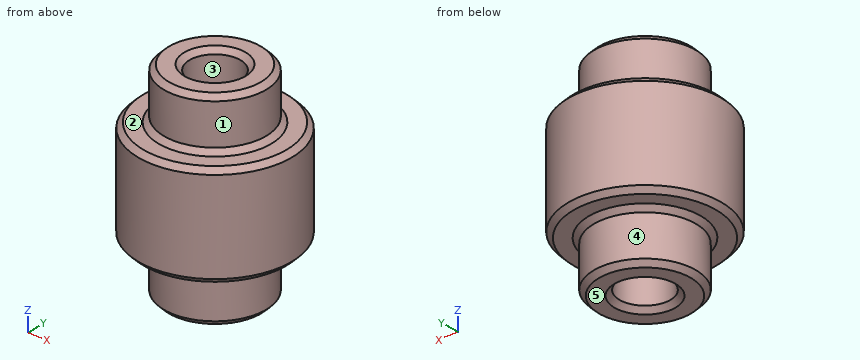
```python
from build123d import *

# Parameters (mm, degrees)
F0_R          = 15
F1_DEPTH      = 10
F1_DEPTH_BACK = 10
F2_R          = 10
F3_DEPTH      = 10
F4_R          = 10
F5_DEPTH      = 10
F7_D          = 10
F8_SIZE       = 1


with BuildPart() as f1:
    # F0 (on Top) → F1 (new body, two sides)
    with BuildSketch(Plane.XY) as f1_sk:
        Circle(F0_R)
    extrude(amount=F1_DEPTH)
    extrude(f1_sk.sketch, amount=-F1_DEPTH_BACK)

    # F2 (on face) → F3 (join)
    with BuildSketch(Plane.XY.offset(10)):
        Circle(F2_R)
    extrude(amount=F3_DEPTH)

    # F4 (on face) → F5 (join)
    with BuildSketch(Plane(origin=(0, 0, -10), x_dir=(1, 0, 0), z_dir=(0, 0, -1))):
        Circle(F4_R)
    extrude(amount=F5_DEPTH)

    # F7 (through all)
    with Locations(Plane.XY.offset(20)):
        with Locations((0, 0)):
            Hole(F7_D / 2)

    # F8
    f8_edges = [f1.edges().sort_by_distance(p)[0] for p in [
        (-10, 0, 20),
        (-5, 0, 20),
        (-15, 0, 10),
        (-10, 0, 10),
        (-15, 0, -10),
        (-10, 0, -10),
        (-10, 0, -20),
        (-5, 0, -20),
    ]]
    chamfer(f8_edges, length=F8_SIZE)


solid = f1.part
```
Can you work these out from the model? Positions are in its coordinate system, mm. Face numbers are marked on the shaded views. A direction names the side the tool comes from. Round coordinates to 2 decimals unless told otherwise and drop trailing zeros. Loops run counter-clockwise (first coordinate to the right, second up) from the corner with the lowest first, then second, coordinate; pieces in that order, holes last.
Item 1: Please list where these lines run through material, in increasing order: L1, parallel to Y at x = 0, z = 8; L2, parallel to Z at x = -5.25, y = -11.5; L3, parallel to Y at x = 4, z = 9.
Item 2: If we mould it in two halves opening along X, with no side actions, what happens to the marked faces 1, 2 and 3? For each: +X half, -X half, draft (parallel to the pull), parting line (faces both ways), or undercut.
Item 3: Suppose I cut it at C-C, the plane z = 4. Write out the boundary of the cut face in (x, y).
Item 4: Suppose I cut it at D-D, the plane z = 13. Write out the boundary of the cut face in (x, y), then the cut area to 3 significant figures.
Item 5: Will these pins go through, and if not, where does the flat tip stop? pin 1 Ø1 at (y, z) = (-6, -2.5) entering from +X; pin 2 Ø4 at (y, z) = (4.5, 14) entering from +X; pin 3 Ø4 at (y, z) = (11.5, -6.5) entering from +X.
Item 6: Which directions (+Z, -Z, +X, -X, +Y, -Y) give clear straight access to the entire face, cutting with the end or side of a thin tool? Please do the marked faces 4 and 5.
Reported:
1. L1: y = -15 to -5, 5 to 15
1. L2: z = -10 to 10
1. L3: y = -14.46 to -3, 3 to 14.46
2. face 1: parting line
2. face 2: draft
2. face 3: undercut
3. outline: circle Ø30 at (0, 0); hole circle Ø10 at (0, 0)
4. outline: circle Ø20 at (0, 0); hole circle Ø10 at (0, 0)
4. area: 236 mm2
5. pin 1: stops at x = 13.96
5. pin 2: stops at x = 9.68
5. pin 3: stops at x = 11.61
6. face 4: -Z
6. face 5: -Z, +X, -X, +Y, -Y
